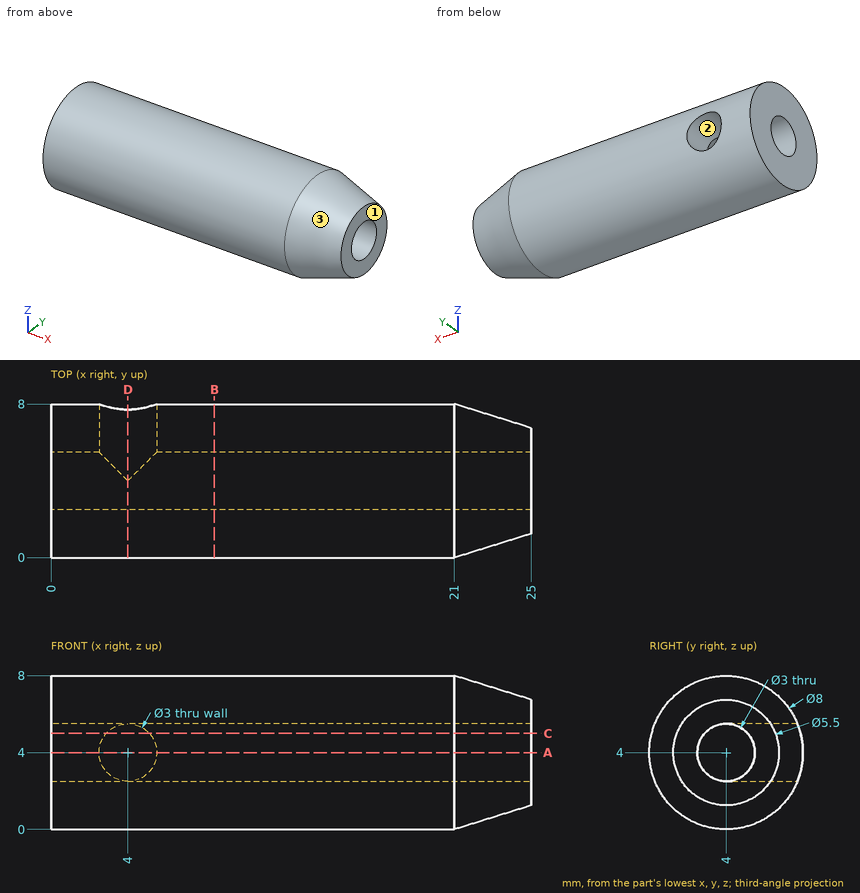
Verification items for this drawing (mm, ordinates from the low corner). Coordinates: 2 decimals unless noted, no trailing zeros. Write each loop counter-clockwise with the first axis right and the second up, starting at its lowest first coordinate (ties: lowest second). Pieces come first, ordered by that corner, then holes. Notation, with made-up numbers: (-31, 24) -> (-7, 24) arc R20 cw to (-7, 46) -> close; hole circle Ø8 at (-21, 51.25). An arc over 180 degrees is marked (long way). Use CSV: the item, a comma, the result in double quotes. Start each with the question number.
Item 1: Cross-section at D-D, the plane x = 4. Record the cut outline in (y, z), plus the area to 3 significant figures.
Item 2: Cross-section at A-A, the plane z = 4. Record the cut outline in (x, y), plus the area to 4 significant figures.
Item 3: Cross-section at B-B, the plane x = 8.5. Record the cut outline in (y, z), plus the area to 3 significant figures.
Item 4: Thickness scan on line 1 (Y direction, x = 16.5, z = 4); line 2 (X direction, y = 6.4, z = 4); line 3 (X direction, y = 5.5, z = 2.75). Record the ranges inside material, lowest first.
Item 5: Mould release check, pull along Z, two halves, no side actions. Record for the marked faces 1, 2 and 3: released by +Z, released by -Z, zero draft, split by the parting line, or undercut.
Item 6: Cross-section at C-C, the plane z = 5. State how many separate pieces and enclosed holes the cut face has, plus the area to 3 significant figures.
Item 7: Depth check by flat-ended pin: pin 1 Ø3.5 at (y, z) = (4, 4) entering from +X; pin 2 Ø2 at (x, y) = (21.5, 5) entering from +Z; pin 3 Ø3 at (x, y) = (22.5, 5.5) entering from +Z. Enter the tip coordinate at first touch or a pass-through.
Answers:
1,outline,"(4, 2.5) arc R1.5 cw to (4, 5.5) -> (7.71, 5.5) arc R4 ccw (long way) to (7.71, 2.5) -> close"
1,area,"35.0 mm^2"
2,outline,"(0, 0) -> (21, 0) -> (25, 1.25) -> (25, 2.5) -> (0, 2.5) -> close; (0, 5.5) -> (2.5, 5.5) -> (2.5, 8) -> (0, 8) -> close; (5.5, 5.5) -> (25, 5.5) -> (25, 6.75) -> (21, 8) -> (5.5, 8) -> close"
2,area,"112.5 mm^2"
3,outline,"circle Ø8 at (4, 4); hole circle Ø3 at (4, 4)"
3,area,"43.2 mm^2"
4,line 1,"0 to 2.5, 5.5 to 8"
4,line 2,"0 to 2.5, 5.5 to 25"
4,line 3,"0 to 3.17, 4.83 to 25"
5,face 1,"zero draft"
5,face 2,"undercut"
5,face 3,"split by the parting line"
6,separate pieces,"3"
6,enclosed holes,"0"
6,area,"126 mm^2"
7,pin 1,"x = 25"
7,pin 2,"z = 8"
7,pin 3,"z = 7.87"
